```python
from build123d import *

# Parameters (mm, degrees)
BOSS_EXTRUDE1_DEPTH = 10
SKETCH2_R           = 2
CUT_EXTRUDE1_DEPTH  = 19
SKETCH3_R           = 1.5
CUT_EXTRUDE2_DEPTH  = 18


with BuildPart() as part:
    # Sketch1 → Boss-Extrude1 (new body)
    with BuildSketch(Plane(origin=(0, 0, 0), x_dir=(1, 0, 0), z_dir=(0, 1, 0))):
        with BuildLine():
            Line((0, 20), (0, 0))
            Line((0, 0), (10, 0))
            Line((10, 0), (10, 8.677124344))
            ThreePointArc((10, 8.677124344), (9.5, 10), (10, 11.322875656))
            Line((10, 11.322875656), (10, 20))
            Line((10, 20), (0, 20))
        make_face()
    extrude(amount=BOSS_EXTRUDE1_DEPTH)

    # Sketch2 → Cut-Extrude1 (cut)
    with BuildSketch(Plane(origin=(10, 0, 0), x_dir=(0, 0, -1), z_dir=(1, 0, 0))):
        with Locations((4, 5)):
            Circle(SKETCH2_R)
        with Locations((16, 5)):
            Circle(SKETCH2_R)
    extrude(amount=-CUT_EXTRUDE1_DEPTH, mode=Mode.SUBTRACT)

    # Sketch3 → Cut-Extrude2 (cut)
    with BuildSketch(Plane(origin=(0, 10, 0), x_dir=(1, 0, 0), z_dir=(0, 1, 0))):
        with Locations(Location((5, 10, 0), (0, 0, 270))):
            Circle(SKETCH3_R)
    extrude(amount=-CUT_EXTRUDE2_DEPTH, mode=Mode.SUBTRACT)


solid = part.part
```
Can you work these out from the model? Positions are in its coordinate system, mm. Coordinates: 2 decimals unless noted, no trailing zeros. Loops run counter-clockwise (first coordinate to the right, second up) from the corner with the lowest first, then second, coordinate; pieces in that order, holes last. Notation, with made-up numbers: (-35, -38.5) -> (21, -38.5) arc R31 ccw to (21, 0.5) -> close; hole circle Ø11 at (1.5, -29.75). An arc over 180 degrees is marked (long way). Answer as a JSON object with one key per item and string values.
1) Imagine slicing it at D-D (y = 7.5). Please give me the cut outline in (x, z).
Results:
{"outline": "(0, -20) -> (10, -20) -> (10, -11.32) arc R2 cw to (10, -8.68) -> (10, 0) -> (0, 0) -> close; hole circle Ø3 at (5, -10)"}
2) Thinking about a two-plate mould opening in Y: for faces 1 (the face through (5, 5, -14)), 2 (the face through (5, 5, 0)), 3 (the face through (7, 0, -10)), which applies, pulls with the +Y half, pulls with the -Y half, needs draft (parallel to the pull), parting line crosses it, or undercut?
Results:
{"face 1": "undercut", "face 2": "needs draft", "face 3": "pulls with the -Y half"}
3) Imagine slicing it at B-B (z = -16). Please give me the cut outline in (x, y).
Results:
{"outline": "(0, 0) -> (10, 0) -> (10, 3) -> (0, 3) -> close; (0, 7) -> (10, 7) -> (10, 10) -> (0, 10) -> close"}
4) Imagine slicing it at A-A (y = 5). Please give me the cut outline in (x, z).
Results:
{"outline": "(0, -20) -> (10, -20) -> (10, -18) -> (0, -18) -> close; (0, -14) -> (10, -14) -> (10, -11.32) arc R2 cw to (10, -8.68) -> (10, -6) -> (0, -6) -> close; (0, -2) -> (10, -2) -> (10, 0) -> (0, 0) -> close; hole circle Ø3 at (5, -10)"}
5) Imagine slicing it at C-C (x = 3). Please give me the cut outline in (y, z), then the cut area to 3 significant figures.
Results:
{"outline": "(0, -20) -> (10, -20) -> (10, 0) -> (0, 0) -> close; hole circle Ø4 at (5, -16); hole circle Ø4 at (5, -4)", "area": "175 mm^2"}
6) If I drill on line 1 (X direction, y = 5.75, z = -10); line 2 (Y direction, x = 3.25, z = -16); line 3 (Y direction, x = 6, z = -17.5), over which ranges is the centre line in solid material (lowest first)?
Results:
{"line 1": "x = 0 to 3.5, 6.5 to 9.5", "line 2": "y = 0 to 3, 7 to 10", "line 3": "y = 0 to 3.68, 6.32 to 10"}
7) For P1, Ø2.5, axis at y = 5, z = -4, coming from the -X side, with a flat end and sliding along its axis, tell me the tip position at first contact or that it passes through.
Results:
{"P1": "passes through"}
